Input: part model. Units: mm. Frame: model coordinates. Face numbers are marked on the shaded views. Round coordinates to 2 decimals unless told otherwise and drop trailing zeros. Order: outer loops, then holes, each group sorted by start corner. A loop starts at its lowest first (then second) coordinate and runs counter-clockwise, first axis right, second up. Notation, with made-up numbers: (59.25, 62.5) -> (67.25, 62.5) arc R21 ccw to (67.25, 76.5) -> close; hole circle Ø4 at (57, 19.25). An arc over 180 degrees is marked (long way). Use a Markdown table: item, result.
from build123d import *

# Parameters (mm, degrees)
F0_W     = 151.980818
F0_H     = 151.646004
F1_DEPTH = 76.2
F2_R     = 32.674685
F3_DEPTH = 151.647003


with BuildPart() as f1:
    # F0 (on Front) → F1 (new body, symmetric)
    with BuildSketch(Plane.XZ):
        Rectangle(F0_W, F0_H)
    extrude(amount=F1_DEPTH, both=True)

    # F2 (on face) → F3 (cut, through all)
    with BuildSketch(Plane(origin=(0, 0, -75.823002), x_dir=(1, 0, 0), z_dir=(0, 0, -1))):
        Circle(F2_R)
    extrude(amount=-F3_DEPTH, mode=Mode.SUBTRACT)


solid = f1.part
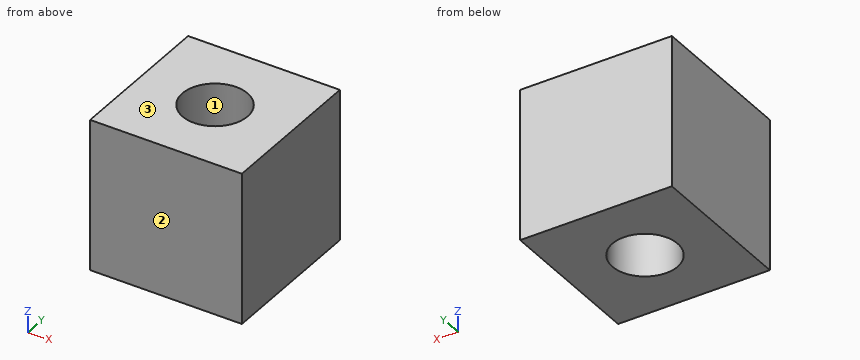
1) Cut plane A-A on x = 0. Return loops of the section in (y, z).
Answer key:
| item | result |
|---|---|
| outline | (-76.2, -75.82) -> (-32.67, -75.82) -> (-32.67, 75.82) -> (-76.2, 75.82) -> close; (32.67, -75.82) -> (76.2, -75.82) -> (76.2, 75.82) -> (32.67, 75.82) -> close |
2) Cut plane C-C on z = 45. Return loops of the section in (x, y), and give its area (3 significant figures).
Answer key:
| item | result |
|---|---|
| outline | (-75.99, -76.2) -> (75.99, -76.2) -> (75.99, 76.2) -> (-75.99, 76.2) -> close; hole circle Ø65.35 at (0, 0) |
| area | 19,800 mm^2 |
3) Cut plane B-B on y = 18. Return loops of the section in (x, z).
Answer key:
| item | result |
|---|---|
| outline | (-75.99, -75.82) -> (-27.27, -75.82) -> (-27.27, 75.82) -> (-75.99, 75.82) -> close; (27.27, -75.82) -> (75.99, -75.82) -> (75.99, 75.82) -> (27.27, 75.82) -> close |
4) Ray query, probe 1 along X at (y, z) = (0, 5); probe 2 along Y at (x, z) = (0, -19.5); probe 3 along X at (y, z) = (-23, -13.5). Return the intervals inside material, ascending.
Answer key:
| item | result |
|---|---|
| probe 1 | x = -75.99 to -32.67, 32.67 to 75.99 |
| probe 2 | y = -76.2 to -32.67, 32.67 to 76.2 |
| probe 3 | x = -75.99 to -23.21, 23.21 to 75.99 |
5) Draft query along Y for the marked faces 1, 2 and 3. Return one class per face: released by +Y, released by -Y, zero draft, split by the parting line, or undercut.
Answer key:
| item | result |
|---|---|
| face 1 | undercut |
| face 2 | released by -Y |
| face 3 | zero draft |
